from build123d import *

# Parameters (mm, degrees)
SKETCH1_R           = 1.6
SKETCH1_R_2         = 1
SKETCH1_R_3         = 5.5
SKETCH1_R_4         = 4.5
BOSS_EXTRUDE2_DEPTH = 2
BOSS_EXTRUDE3_START = -2
SKETCH2_R           = 1
BOSS_EXTRUDE3_DEPTH = 2
SKETCH3_R           = 1
CUT_EXTRUDE1_DEPTH  = 103
BOSS_EXTRUDE4_START = -2
SKETCH4_R           = 1.6
BOSS_EXTRUDE4_DEPTH = 2
SKETCH5_R           = 1.6
CUT_EXTRUDE2_DEPTH  = 10
SKETCH6_R           = 1.6
CUT_EXTRUDE3_DEPTH  = 10
BOSS_EXTRUDE5_DEPTH = 2
CUT_EXTRUDE4_DEPTH  = 10
SKETCH10_R          = 1.6
SKETCH10_R_2        = 5.5
SKETCH10_R_3        = 4.5
BOSS_EXTRUDE6_DEPTH = 2
FILLET2_START       = -1
FILLET2_DEPTH       = 4
FILLET2_2_DEPTH     = 2


with BuildPart() as part:
    # Sketch1 → Boss-Extrude2 (new body)
    with BuildSketch(Plane(origin=(0, 0, 0), x_dir=(1, 0, 0), z_dir=(0, 1, 0))):
        with BuildLine():
            Line((12.313589515, -16.493996637), (35.979225245, -12.848450001))
            ThreePointArc((35.979225245, -12.848450001), (46.993067566, -0.424494085), (36.813648041, 12.691862933))
            Line((36.813648041, 12.691862933), (35.165189196, 12.947676785))
            Line((35.165189196, 12.947676785), (12.319067304, 16.493021261))
            ThreePointArc((12.319067304, 16.493021261), (11.720527595, 16.549330191), (11.119556233, 16.533395936))
            Line((11.119556233, 16.533395936), (-11.812019178, 14.541098507))
            ThreePointArc((-11.812019178, 14.541098507), (-13.247239988, 14.027709898), (-14.244912332, 12.87528787))
            Line((-14.244912332, 12.87528787), (-19.487592157, 2.204884721))
            ThreePointArc((-19.487592157, 2.204884721), (-19.693653105, -1.723258696), (-16.994761113, -4.584858569))
            Line((-16.994761113, -4.584858569), (9.557587922, -16.137143667))
            ThreePointArc((9.557587922, -16.137143667), (10.910298182, -16.51089082), (12.313589515, -16.493996637))
        make_face()
        with Locations(Location((11.552349036, -11.552285098, 0), (0, 0, 270))):
            Circle(SKETCH1_R, mode=Mode.SUBTRACT)
        with Locations(Location((25, -11, 0), (0, 0, 270))):
            Circle(SKETCH1_R_2, mode=Mode.SUBTRACT)
        with Locations(Location((-15, 0, 0), (0, 0, 270))):
            Circle(SKETCH1_R, mode=Mode.SUBTRACT)
        with Locations(Location((0, 0, 0), (0, 0, 270))):
            Circle(SKETCH1_R_3, mode=Mode.SUBTRACT)
        with Locations(Location((-11.552357038, 11.552357038, 0), (0, 0, 270))):
            Circle(SKETCH1_R, mode=Mode.SUBTRACT)
        with Locations(Location((11.552326466, 11.552160153, 0), (0, 0, 270))):
            Circle(SKETCH1_R, mode=Mode.SUBTRACT)
        with Locations(Location((14, 0, 0), (0, 0, 270))):
            Circle(SKETCH1_R_4, mode=Mode.SUBTRACT)
        with Locations(Location((34, 0, 0), (0, 0, 270))):
            Circle(SKETCH1_R_4, mode=Mode.SUBTRACT)
        with Locations(Location((25, 11, 0), (0, 0, 270))):
            Circle(SKETCH1_R_2, mode=Mode.SUBTRACT)
    extrude(amount=BOSS_EXTRUDE2_DEPTH)

    # Sketch2 → Boss-Extrude3 (add)
    with BuildSketch(Plane(origin=(0, 2, 0), x_dir=(1, 0, 0), z_dir=(0, 1, 0)).offset(BOSS_EXTRUDE3_START)):
        with Locations((25, 11)):
            Circle(SKETCH2_R)
        with Locations((25, -11)):
            Circle(SKETCH2_R)
    extrude(amount=BOSS_EXTRUDE3_DEPTH)

    # Sketch3 → Cut-Extrude1 (cut)
    with BuildSketch(Plane(origin=(0, 2, 0), x_dir=(1, 0, 0), z_dir=(0, 1, 0))):
        with Locations(Location((24, 13, 0), (0, 0, 270))):
            Circle(SKETCH3_R)
        with Locations(Location((24, -13, 0), (0, 0, 270))):
            Circle(SKETCH3_R)
    extrude(amount=-CUT_EXTRUDE1_DEPTH, mode=Mode.SUBTRACT)

    # Sketch4 → Boss-Extrude4 (add)
    with BuildSketch(Plane(origin=(0, 2, 0), x_dir=(1, 0, 0), z_dir=(0, 1, 0)).offset(BOSS_EXTRUDE4_START)):
        with Locations((-11.552357038, 11.552357038)):
            Circle(SKETCH4_R)
        with Locations((11.552326466, 11.552160153)):
            Circle(SKETCH4_R)
        with Locations((11.552349036, -11.552285098)):
            Circle(SKETCH4_R)
    extrude(amount=BOSS_EXTRUDE4_DEPTH)

    # Sketch5 → Cut-Extrude2 (cut)
    with BuildSketch(Plane(origin=(0, 2, 0), x_dir=(1, 0, 0), z_dir=(0, 1, 0))):
        with Locations(Location((-11.66726189, 11.66726189, 0), (0, 0, 270))):
            Circle(SKETCH5_R)
        with Locations(Location((11.66726189, 11.66726189, 0), (0, 0, 270))):
            Circle(SKETCH5_R)
        with Locations(Location((11.66726189, -11.66726189, 0), (0, 0, 270))):
            Circle(SKETCH5_R)
    extrude(amount=-CUT_EXTRUDE2_DEPTH, mode=Mode.SUBTRACT)

    # Sketch6 → Cut-Extrude3 (cut)
    with BuildSketch(Plane(origin=(0, 2, 0), x_dir=(1, 0, 0), z_dir=(0, 1, 0))):
        with Locations((24, 12.25)):
            Circle(SKETCH6_R)
        with Locations((24, -12.25)):
            Circle(SKETCH6_R)
    extrude(amount=-CUT_EXTRUDE3_DEPTH, mode=Mode.SUBTRACT)

    # Sketch7 → Boss-Extrude5 (add)
    with BuildSketch(Plane(origin=(0, 2, 0), x_dir=(1, 0, 0), z_dir=(0, 1, 0))):
        with BuildLine():
            ThreePointArc((24.746843357, 13.665), (24, 14), (23.253156643, 13.665))
            ThreePointArc((23.253156643, 13.665), (24, 13.85), (24.746843357, 13.665))
        make_face()
        with BuildLine():
            ThreePointArc((23.253156643, -13.665), (24, -13.85), (24.746843357, -13.665))
            ThreePointArc((24.746843357, -13.665), (24, -14), (23.253156643, -13.665))
        make_face()
    extrude(amount=-BOSS_EXTRUDE5_DEPTH)

    # Sketch8 → Cut-Extrude4 (cut)
    with BuildSketch(Plane(origin=(0, 2, 0), x_dir=(1, 0, 0), z_dir=(0, 1, 0))):
        with BuildLine():
            Line((-14.308416207, 12.704426351), (-18.723213135, 1.462082061))
            ThreePointArc((-18.723213135, 1.462082061), (-16.986293656, -3.471978904), (-11.852582747, -2.468555172))
            Line((-11.852582747, -2.468555172), (6.930322315, -10.68631196))
            ThreePointArc((6.930322315, -10.68631196), (7.786759617, -14.555611143), (11.247508844, -16.486459611))
            Line((11.247508844, -16.486459611), (11.232461738, -16.659215907))
            Line((11.232461738, -16.659215907), (-9.768707716, -29.444072038))
            Line((-9.768707716, -29.444072038), (-31.03313029, 2.888905984))
            Line((-31.03313029, 2.888905984), (-14.308416207, 12.704426351))
        make_face()
    extrude(amount=-CUT_EXTRUDE4_DEPTH, mode=Mode.SUBTRACT)

    # Sketch10 → Boss-Extrude6 (add)
    # profile 1 of 3: a face of its own
    with BuildSketch(Plane(origin=(0, 2, 0), x_dir=(1, 0, 0), z_dir=(0, 1, 0))):
        with BuildLine():
            Line((6.930322315, -10.68631196), (-2.461130216, -6.577433566))
            Line((-2.461130216, -6.577433566), (-2.861958704, -7.493586677))
            Line((-2.861958704, -7.493586677), (6.830279674, -11.734062656))
            ThreePointArc((6.830279674, -11.734062656), (6.851720384, -11.207458338), (6.930322315, -10.68631196))
        make_face()
    # profile 2 of 3: a face of its own
    with BuildSketch(Plane(origin=(0, 2, 0), x_dir=(1, 0, 0), z_dir=(0, 1, 0))):
        with BuildLine():
            Line((-2.861958704, -7.493586677), (-2.461130216, -6.577433566))
            Line((-2.461130216, -6.577433566), (-11.852582747, -2.468555172))
            ThreePointArc((-11.852582747, -2.468555172), (-12.214781898, -2.870985915), (-12.628009506, -3.220816837))
            Line((-12.628009506, -3.220816837), (-2.861958704, -7.493586677))
        make_face()
    # profile 3 of 3: a face of its own
    with BuildSketch(Plane(origin=(0, 2, 0), x_dir=(1, 0, 0), z_dir=(0, 1, 0))):
        with BuildLine():
            Line((8.035421862, -12.261327493), (6.830279674, -11.734062656))
            ThreePointArc((6.830279674, -11.734062656), (8.124009767, -14.960622436), (11.247508844, -16.486459611))
            Line((11.247508844, -16.486459611), (11.242611849, -16.542682164))
            ThreePointArc((11.242611849, -16.542682164), (11.779409327, -16.5471268), (12.313589515, -16.493996637))
            Line((12.313589515, -16.493996637), (35.979225245, -12.848450001))
            ThreePointArc((35.979225245, -12.848450001), (46.993067566, -0.424494085), (36.813648041, 12.691862933))
            Line((36.813648041, 12.691862933), (12.319067304, 16.493021261))
            ThreePointArc((12.319067304, 16.493021261), (11.720527595, 16.549330191), (11.119556233, 16.533395936))
            Line((11.119556233, 16.533395936), (-11.812019178, 14.541098507))
            ThreePointArc((-11.812019178, 14.541098507), (-13.247239988, 14.027709898), (-14.244912332, 12.87528787))
            Line((-14.244912332, 12.87528787), (-14.337145922, 12.68756525))
            Line((-14.337145922, 12.68756525), (-14.308416207, 12.704426351))
            Line((-14.308416207, 12.704426351), (-18.723213135, 1.462082061))
            ThreePointArc((-18.723213135, 1.462082061), (-17.436972748, -3.171933767), (-12.628009506, -3.220816837))
            Line((-12.628009506, -3.220816837), (-13.301998386, -2.925938239))
            Line((-13.301998386, -2.925938239), (-11.820094843, -1.440006983))
            Line((-11.820094843, -1.440006983), (-1.105948659, -6.127580457))
            Line((-1.105948659, -6.127580457), (8.611687481, -8.831618339))
            Line((8.611687481, -8.831618339), (8.035421862, -12.261327493))
        make_face()
        with Locations(Location((11.66726189, -11.66726189, 0), (0, 0, 270))):
            Circle(SKETCH10_R, mode=Mode.SUBTRACT)
        with Locations(Location((24, -12.25, 0), (0, 0, 270))):
            Circle(SKETCH10_R, mode=Mode.SUBTRACT)
        with Locations(Location((-15, 0, 0), (0, 0, 270))):
            Circle(SKETCH10_R, mode=Mode.SUBTRACT)
        with Locations(Location((0, 0, 0), (0, 0, 270))):
            Circle(SKETCH10_R_2, mode=Mode.SUBTRACT)
        with Locations(Location((-11.66726189, 11.66726189, 0), (0, 0, 270))):
            Circle(SKETCH10_R, mode=Mode.SUBTRACT)
        with Locations(Location((11.66726189, 11.66726189, 0), (0, 0, 270))):
            Circle(SKETCH10_R, mode=Mode.SUBTRACT)
        with Locations(Location((14, 0, 0), (0, 0, 270))):
            Circle(SKETCH10_R_3, mode=Mode.SUBTRACT)
        with Locations(Location((34, 0, 0), (0, 0, 270))):
            Circle(SKETCH10_R_3, mode=Mode.SUBTRACT)
        with Locations(Location((24, 12.25, 0), (0, 0, 270))):
            Circle(SKETCH10_R, mode=Mode.SUBTRACT)
    extrude(amount=-BOSS_EXTRUDE6_DEPTH)

    # Fillet2: read off the stored shape, not the designer's step
    # Fillet2 outline → Fillet2 (cut)
    with BuildSketch(Plane(origin=(0, 0, 0), x_dir=(1, 0, 0), z_dir=(0, 1, 0)).offset(FILLET2_START)):
        with BuildLine():
            ThreePointArc((11.242611849, -16.542682164), (11.704154362, -16.549980081), (12.16440304, -16.514682694))
            ThreePointArc((12.16440304, -16.514682694), (11.70487082, -16.535823924), (11.247508844, -16.486459611))
            Line((11.247508844, -16.486459611), (11.242611849, -16.542682164))
        make_face()
    extrude(amount=FILLET2_DEPTH, mode=Mode.SUBTRACT)

    # Fillet2 2 outline → Fillet2 2 (add)
    with BuildSketch(Plane(origin=(0, 0, 0), x_dir=(1, 0, 0), z_dir=(0, 1, 0))):
        with BuildLine():
            ThreePointArc((-13.580529798, -3.739666341), (-12.441461916, -3.545340418), (-11.313441681, -3.795956765))
            Line((-11.313441681, -3.795956765), (-12.628009506, -3.220816837))
            ThreePointArc((-12.628009506, -3.220816837), (-13.086601256, -3.512677788), (-13.580529798, -3.739666341))
        make_face()
        with BuildLine():
            ThreePointArc((5.336294885, -11.080425553), (6.391396593, -11.853207748), (7.01744839, -13.001463417))
            ThreePointArc((7.01744839, -13.001463417), (6.88172123, -12.373986651), (6.830279674, -11.734062656))
            Line((6.830279674, -11.734062656), (5.336294885, -11.080425553))
        make_face()
    extrude(amount=FILLET2_2_DEPTH)


solid = part.part
Verification items for the finished model (mm, model axes). Give positions to 0.01 mm unless a question says otherwise; leave off trailing zeros. Write each loop counter-clockwise with the first axis right and the second up, starting at its lowest first coordinate (ties: lowest second). Pieces come first, ordered by that corner, then holes. Notation, with made-up numbers: (-12.75, -33.75) - (9.25, -33.75) arc R19 ccw to (9.25, -1.75) - close; hole circle Ø8 at (-12, 32). An arc over 180 degrees is marked (long way). Answer as CSV lines item,"result". Start each with the question number.
1. Sectioned sample at B-B (x = 1). Record the boundary of the cut face in (y, z), then the cut area to 3 significant figures.
2. Draft check along Z on faces 1 (the face through (-5.37, 0.99, -1.19)), 2 (the face through (6.38, 0.99, 11.84)), 3 (the face through (13.02, 1.01, -10.81)), 4 (the face through (11.73, 0.99, -16.55)). Enter one of: pulls with the +Z half, pulls with the -Z half, needs draft (parallel to the pull), parting line crosses it, or undercut.
3. Depth check by flat-ended pin: pin 1 (10.5 mm diameter, centred on x = 34, z = 0, fed in from -Y). Enter the tip coordinate at first touch or a pass-through.
4. Sectioned sample at D-D (z = 12.25). Record the boundary of the cut face in (x, y).
5. Sectioned sample at A-A (z = 0). Record the boundary of the cut face in (x, y), then the cut area to 3 significant figures.
6. Thickness scan on line 1 (X direction, y = 1.2, z = 0); line 2 (Z direction, x = 23.5, y = 1.7); line 3 (X direction, y = 1.75, z = -11.5). Record the ranges inside material, lowest first.
7. Sectioned sample at C-C (y = 1.6). Count the separate pieces of the cut face and the enclosed holes in it, then the cut area to 3 significant figures.
Derived:
1,outline,"(0, -15.65) - (2, -15.65) - (2, -5.41) - (0, -5.41) - close; (0, 5.41) - (2, 5.41) - (2, 9.18) - (0, 9.18) - close"
1,area,"28.0 mm²"
2,face 1,"undercut"
2,face 2,"pulls with the +Z half"
2,face 3,"undercut"
2,face 4,"pulls with the -Z half"
3,pin 1,"y = 0"
4,outline,"(6.68, 0) - (10.18, 0) - (10.18, 2) - (6.68, 2) - close; (13.16, 0) - (22.4, 0) - (22.4, 2) - (13.16, 2) - close; (25.6, 0) - (38.35, 0) - (38.35, 2) - (25.6, 2) - close"
5,outline,"(-19, 0) - (-16.6, 0) - (-16.6, 2) - (-19, 2) - close; (-13.4, 0) - (-5.5, 0) - (-5.5, 2) - (-13.4, 2) - close; (5.5, 0) - (9.5, 0) - (9.5, 2) - (5.5, 2) - close; (18.5, 0) - (29.5, 0) - (29.5, 2) - (18.5, 2) - close; (38.5, 0) - (47, 0) - (47, 2) - (38.5, 2) - close"
5,area,"67.6 mm²"
6,line 1,"-19 to -16.6, -13.4 to -5.5, 5.5 to 9.5, 18.5 to 29.5, 38.5 to 47"
6,line 2,"-14.76 to -13.77, -10.73 to 10.73, 13.77 to 14.77"
6,line 3,"-14.78 to -13.26, -10.08 to 10.08, 13.26 to 22.59, 25.41 to 40.06"
7,separate pieces,"1"
7,enclosed holes,"9"
7,area,"1,330 mm²"
